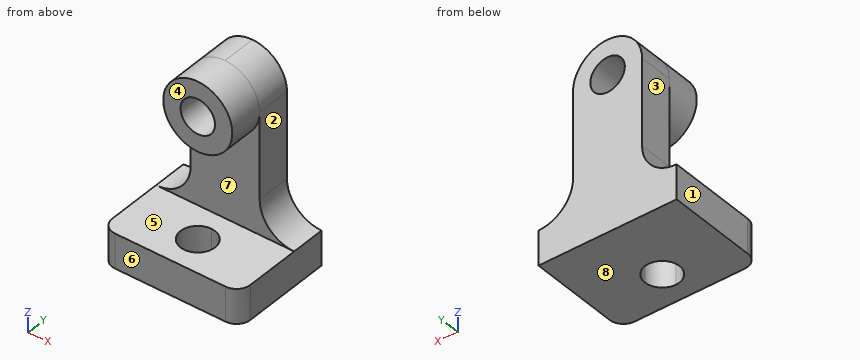
```python
from build123d import *

# Parameters (mm, degrees)
F0_W      = 12.7
F0_H      = 12.7
F1_DEPTH  = 12.7
F3_DEPTH  = 25.4
F4_W      = 50.8
F4_H      = 12.7
F5_DEPTH  = 25.4
F6_R      = 5.08
F7_R      = 12.7
F7_R_2    = 6.35
F8_DEPTH  = 12.7
F9_DEPTH  = 25.4
F11_DEPTH = 25.4


with BuildPart() as f1:
    # F0 (on Front) → F1 (new body)
    with BuildSketch(Plane.XZ):
        with BuildLine():
            Line((0, 31.75), (0, 0))
            Line((0, 0), (12.7, 0))
            Line((12.7, 0), (12.7, 12.7))
            Line((12.7, 12.7), (12.7, 44.45))
            ThreePointArc((12.7, 44.45), (8.9802561211, 35.4697438789), (0, 31.75))
        make_face()
        Polygon((12.7, 0), (0, 0), (-12.7, 0), (-25.4, 0), (-25.4, -12.7), (0, -12.7), (25.4, -12.7), (25.4, 0), align=None)
        with BuildLine():
            Line((-12.7, 0), (0, 0))
            Line((0, 0), (0, 31.75))
            ThreePointArc((0, 31.75), (-8.9802561211, 35.4697438789), (-12.7, 44.45))
            Line((-12.7, 44.45), (-12.7, 12.7))
            Line((-12.7, 12.7), (-12.7, 0))
        make_face()
        with Locations((19.05, 6.35)):
            Rectangle(F0_W, F0_H)
        with Locations((-19.05, 6.35)):
            Rectangle(F0_W, F0_H)
        with BuildLine():
            ThreePointArc((-12.7, 44.45), (-8.9802561211, 35.4697438789), (0, 31.75))
            Line((0, 31.75), (0, 44.45))
            Line((0, 44.45), (-12.7, 44.45))
        make_face()
        with BuildLine():
            Line((0, 44.45), (0, 31.75))
            ThreePointArc((0, 31.75), (8.9802561211, 35.4697438789), (12.7, 44.45))
            Line((12.7, 44.45), (0, 44.45))
        make_face()
        with BuildLine():
            Line((-12.7, 44.45), (0, 44.45))
            Line((0, 44.45), (0, 57.15))
            ThreePointArc((0, 57.15), (-8.9802561211, 53.4302561211), (-12.7, 44.45))
        make_face()
        with BuildLine():
            Line((0, 57.15), (0, 44.45))
            Line((0, 44.45), (12.7, 44.45))
            ThreePointArc((12.7, 44.45), (8.9802561211, 53.4302561211), (0, 57.15))
        make_face()
    extrude(amount=F1_DEPTH)

    # F2 (on face) → F3 (cut)
    with BuildSketch(Plane(origin=(0, 0, 0), x_dir=(-1, 0, 0), z_dir=(0, 1, 0))):
        with BuildLine():
            Line((25.4, 12.7), (12.7, 12.7))
            ThreePointArc((12.7, 12.7), (16.4197438789, 3.7197438789), (25.4, 0))
            Line((25.4, 0), (25.4, 12.7))
        make_face()
        with BuildLine():
            ThreePointArc((-25.4, 0), (-16.4197438789, 3.7197438789), (-12.7, 12.7))
            Line((-12.7, 12.7), (-25.4, 12.7))
            Line((-25.4, 12.7), (-25.4, 0))
        make_face()
    extrude(amount=-F3_DEPTH, mode=Mode.SUBTRACT)

    # F4 (on face) → F5 (join)
    with BuildSketch(Plane.XZ.offset(12.7)):
        with Locations((0, -6.35)):
            Rectangle(F4_W, F4_H)
    extrude(amount=F5_DEPTH)

    # F6
    f6_edges = [f1.edges().sort_by_distance(p)[0] for p in [
        (25.4, -38.1, -6.35),
        (-25.4, -38.1, -6.35),
    ]]
    fillet(f6_edges, radius=F6_R)

    # F7 (on face) → F8 (join)
    with BuildSketch(Plane.XZ.offset(12.7)):
        with Locations((0, 44.45)):
            Circle(F7_R)
        with Locations((0, 44.45)):
            Circle(F7_R_2, mode=Mode.SUBTRACT)
    extrude(amount=F8_DEPTH)

    # F9 (cut): a face of the model
    f9_faces = [f1.faces().sort_by_distance(p)[0] for p in [
        (0, -12.7, 44.45),
    ]]
    extrude(f9_faces, amount=-F9_DEPTH, mode=Mode.SUBTRACT)

    # F10 (on face) → F11 (cut)
    with BuildSketch(Plane(origin=(0, 0, -12.7), x_dir=(1, 0, 0), z_dir=(0, 0, -1))):
        with BuildLine():
            ThreePointArc((0, 31.75), (-6.35, 25.4), (0, 19.05))
            Line((0, 19.05), (0, 25.4))
            Line((0, 25.4), (0, 31.75))
        make_face()
        with BuildLine():
            Line((0, 25.4), (0, 19.05))
            ThreePointArc((0, 19.05), (4.4901280605, 20.9098719395), (6.35, 25.4))
            ThreePointArc((6.35, 25.4), (4.4901280605, 29.8901280605), (0, 31.75))
            Line((0, 31.75), (0, 25.4))
        make_face()
    extrude(amount=-F11_DEPTH, mode=Mode.SUBTRACT)


solid = f1.part
```
The listing builds one solid part. Answer for the finished solid, in the listing's coordinates (mm). Face numbers are marked on the shaded views. A direction names the side the tool comes from. Round coordinates to 2 decimals unless told otherwise and drop trailing zeros. Order: outer loops, then holes, each group sorted by start corner. A loop starts at its lowest first (then second) coordinate and runs counter-clockwise, first axis right, second up. Notation, with made-up numbers: (30, -14) -> (36, -14) arc R20 ccw to (36, -9) -> close; hole circle Ø8 at (11, -21.5). An arc over 180 degrees is marked (long way). Answer as CSV lines item,"result". Start each with the question number.
(1) For a pull along Z with two mould halves and no side action, classify the marked faces 6, 7 and 8 as +Z half, -Z half, draft (parallel to the pull), parting line (faces both ways), or undercut.
(2) The part is cut by section D-D (x = -1). Determine the outline of the cut face in (y, z).
(3) Find the intervals of material crossed by probe 1 along Z at (x, y) = (0, -16); probe 2 along X at (y, z) = (-10, 44); probe 3 along Z at (x, y) = (0, -21.25), in increasing order. Write a range as from..to.
(4) Flat-ended cylindrical pins translate along their axes: pin 1 Ø1 at (y, z) = (-11, 35) entering from -X; pin 2 Ø14.5 at (x, z) = (0, 44.45) entering from -Y; pin 3 Ø6.5 at (y, z) = (-8, 24.5) entering from +X. Find the tip coordinate at first contact, or state that the pin passes through.
(5) The part is cut by section B-B (z = 49.5). Determine the outline of the cut face in (x, y).
(6) A tool of negligible diameter and unlimited length cuts with its end or side. For the marked faces 1, 2, 3, 4 and 5, from which of +Z, -Z, +X, -X, +Y, -Y can it reach the whole face along a straight path? Write none if from no direction.
(7) The part is cut by section C-C (y = -20). Determine the outline of the cut face in (x, z).
(8) The part is cut by section A-A (y = -5.5). Determine the outline of the cut face in (x, z), then the cut area to 3 significant figures.
Evaluation:
1,face 6,"draft"
1,face 7,"undercut"
1,face 8,"-Z half"
2,outline,"(-38.1, -12.7) -> (-31.67, -12.7) -> (-31.67, 0) -> (-38.1, 0) -> close; (-25.4, 31.79) -> (-12.7, 31.79) -> (-12.7, 0) -> (-19.13, 0) -> (-19.13, -12.7) -> (0, -12.7) -> (0, 38.18) -> (-25.4, 38.18) -> close; (-25.4, 50.72) -> (0, 50.72) -> (0, 57.11) -> (-25.4, 57.11) -> close"
3,probe 1,"-12.7..0, 31.75..38.1, 50.8..57.15"
3,probe 2,"-12.7..-6.33, 6.33..12.7"
3,probe 3,"31.75..38.1, 50.8..57.15"
4,pin 1,"x = -12.7"
4,pin 2,"y = -25.4"
4,pin 3,"x = 12.7"
5,outline,"(-11.65, -25.4) -> (-3.85, -25.4) -> (-3.85, 0) -> (-11.65, 0) -> close; (3.85, -25.4) -> (11.65, -25.4) -> (11.65, 0) -> (3.85, 0) -> close"
6,face 1,"+Z, -Z, -X, +Y, -Y"
6,face 2,"+Z, +X, +Y, -Y"
6,face 3,"+Z, -X, +Y, -Y"
6,face 4,"+Z, +X, -X, -Y"
6,face 5,"+X, -X, -Y"
7,outline,"(-25.4, -12.7) -> (-3.34, -12.7) -> (-3.34, 0) -> (-25.4, 0) -> close; circle Ø25.4 at (0, 44.45); (3.34, -12.7) -> (25.4, -12.7) -> (25.4, 0) -> (3.34, 0) -> close; hole circle Ø12.7 at (0, 44.45)"
8,outline,"(-25.4, -12.7) -> (25.4, -12.7) -> (25.4, 0) arc R12.7 cw to (12.7, 12.7) -> (12.7, 44.45) arc R12.7 ccw to (-12.7, 44.45) -> (-12.7, 12.7) arc R12.7 cw to (-25.4, 0) -> close; hole circle Ø12.7 at (0, 44.45)"
8,area,"1,970 mm²"
